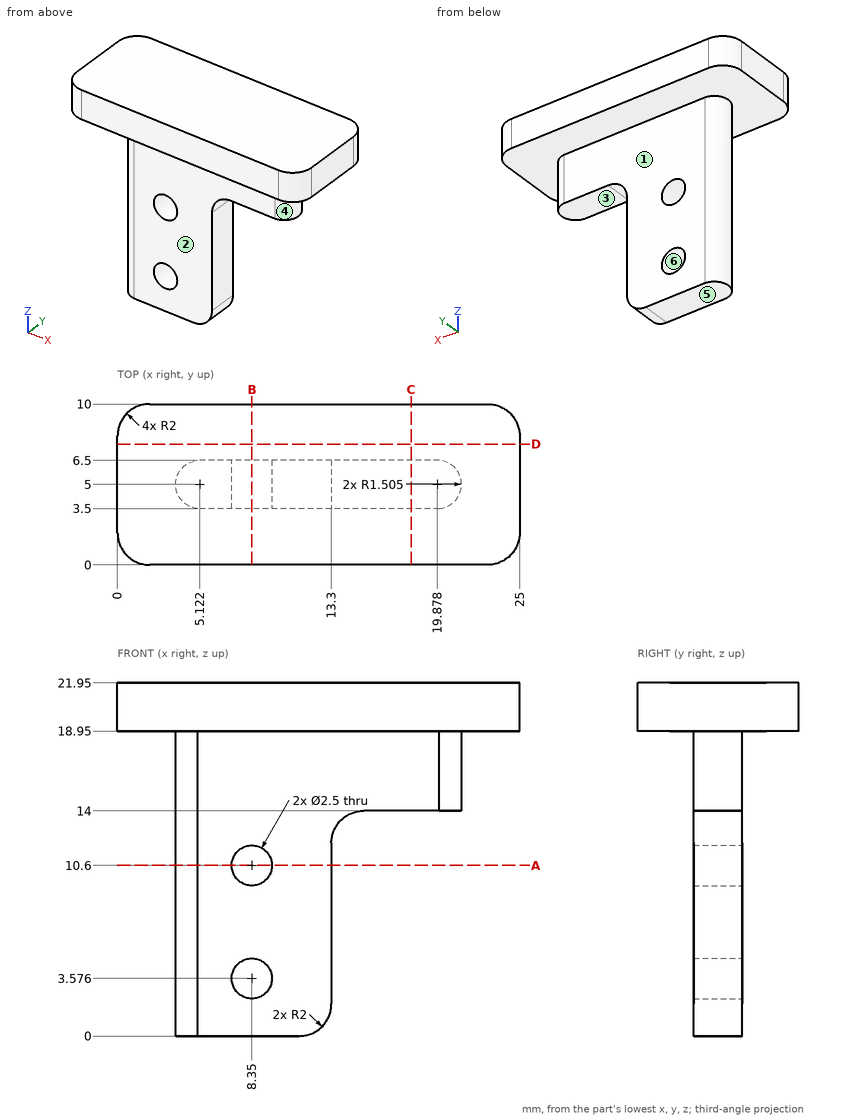
Input: dimensioned drawing with shaded views. Units: mm. Origin: part minimum x, y, z. A direction names the side the tool comes from. Round coordinates to 2 decimals unless told otherwise and drop trailing zeros. Loops run counter-clockwise (first coordinate to the right, second up) from the corner with the lowest first, then second, coordinate; pieces in that order, holes last. Notation, with made-up numbers: (35, -37) -> (61, -37) arc R22 cw to (61, -14) -> close; hole circle Ø4 at (71.25, 38.25). An arc over 180 degrees is marked (long way). Answer as a JSON object with one key per item and string values. Group by question number.
1) Reachability of the marked faces 1, 2 and 3 from +Z, -Z, +X, -X, +Y, -Y: full face, straight path, thin tool, end or side. Return the list, or none.
2) Pin query (flat end, axial travel): pin 1 (3 mm diameter, centred on x = 6, z = 3, fed in from +Y); pin 2 (2 mm diameter, centred on x = 8.35, z = 3.576, fed in from +Y); pin 3 (3.5 mm diameter, centred on x = 18, y = 4.5, fed in from -Z); pin 4 (1.5 mm diameter, centred on y = 5.5, z = 7.5, fed in from +X). Return the tip coordinate at first contact, or that it passes through.
3) Draft query along X for the marked faces 4, 5 and 6. Return one class per face: +X half, -X half, draft (parallel to the pull), parting line (faces both ways), or undercut.
4) Section query C-C on x = 18.25. Output: boundary loops of the cut face in (y, z).
5) Ray query, L1, parallel to Z at x = 8.35, y = 5.6; L2, parallel to X at y = 5.05, z = 10.6; L3, parallel to Y at x = 18.25, z = 18.75. Return the intervals inside material, ascending.
6) Section query D-D on y = 7.5. Output: boundary loops of the cut face in (x, z).
7) Section query B-B on x = 8.35. Output: boundary loops of the cut face in (y, z).
8) Section query A-A on z = 10.6. Output: boundary loops of the cut face in (x, y) (1 decimal), plus the area to 3 significant figures.
Reply:
{
 "1": {"face 1": "-Z, +X, -X, +Y", "face 2": "-Z, +X, -X, -Y", "face 3": "-Z, +X, +Y, -Y"},
 "2": {"pin 1": "stops at y = 6.5", "pin 2": "passes through", "pin 3": "stops at z = 14", "pin 4": "stops at x = 13.3"},
 "3": {"face 4": "+X half", "face 5": "draft", "face 6": "undercut"},
 "4": {"outline": "(0, 18.95) -> (3.5, 18.95) -> (3.5, 14) -> (6.5, 14) -> (6.5, 18.95) -> (10, 18.95) -> (10, 21.95) -> (0, 21.95) -> close"},
 "5": {"L1": "z = 0 to 2.33, 4.83 to 9.35, 11.85 to 21.95", "L2": "x = 3.62 to 7.1, 9.6 to 13.3", "L3": "y = 3.5 to 6.5"},
 "6": {"outline": "(0, 18.95) -> (25, 18.95) -> (25, 21.95) -> (0, 21.95) -> close"},
 "7": {"outline": "(0, 18.95) -> (3.5, 18.95) -> (3.5, 11.85) -> (6.5, 11.85) -> (6.5, 18.95) -> (10, 18.95) -> (10, 21.95) -> (0, 21.95) -> close; (3.5, 0) -> (6.5, 0) -> (6.5, 2.33) -> (3.5, 2.33) -> close; (3.5, 4.83) -> (6.5, 4.83) -> (6.5, 9.35) -> (3.5, 9.35) -> close"},
 "8": {"outline": "(5, 3.5) -> (7.1, 3.5) -> (7.1, 6.5) -> (5, 6.5) arc R1.5 ccw to start; (9.6, 3.5) -> (13.3, 3.5) -> (13.3, 6.5) -> (9.6, 6.5) -> close", "area": "20.6 mm2"}
}
